Autodesk Fusion 360 part; units mm, degrees
sketch "Sketch1" plane through (0, 0, 0) normal (0, 0, 1) x (1, 0, 0)
  line L0 (10, -7.5) -> (-10, -7.5)
  line L1 (-10, -7.5) -> (-10, 7.5)
  line L2 (-10, 7.5) -> (10, 7.5)
  line L3 (10, 7.5) -> (10, -7.5)
  line L4 (10, -7.5) -> (-10, 7.5) construction
  line L5 (-10, -7.5) -> (10, 7.5) construction
  line L6 (0, 0) -> (0, 7) construction
  dimension "d1" = 20
  dimension "d2" = 15
extrude "Extrude1" add sketch "Sketch1" along normal blind 4
sketch "Sketch2" plane through (0, 0, 4) normal (0, 0, 1) x (-1, 0, 0)
  line L0 (-10, -7.5) -> (10, -7.5)
  line L1 (10, -7.5) -> (10, 7.5)
  line L2 (10, 7.5) -> (-10, 7.5)
  line L3 (-10, 7.5) -> (-10, -7.5)
  line L4 (10, 7.5) -> (-10, -7.5) construction
  line L5 (-10, 7.5) -> (10, -7.5) construction
  line L6 (0, 0) -> (-3, 0) construction
  circle A0 centre (-3, 0) radius 1
  line L7 (0, 0) -> (3, 0) construction
  circle A1 centre (3, 0) radius 1
  dimension "d5" = 3
  dimension "d6" = 2
  dimension "d7" = 3
  dimension "d8" = 2
extrude "Extrude2" cut sketch "Sketch2" against normal up to surface (4 mm away) contours A0 | A1
ref_plane "WorkPlane1" through (48, 0, 2) normal (1, 0, 0) x (0, 1, 0)
sketch "Sketch3" plane through (48, 0, 2) normal (1, 0, 0) x (0, 1, 0)
  line L0 (-7.5, 2) -> (-2.5, 2)
  line L1 (-2.5, 2) -> (-2.5, -2)
  line L2 (-2.5, -2) -> (-7.5, -2)
  line L3 (-7.5, -2) -> (-7.5, 2)
  line L4 (7.5, 2) -> (2.5, 2)
  line L5 (2.5, 2) -> (2.5, -2)
  line L6 (2.5, -2) -> (7.5, -2)
  line L7 (7.5, -2) -> (7.5, 2)
extrude "Extrude3" add sketch "Sketch3" against normal up to surface (38 mm away)
sketch "Sketch4" plane through (0, -2.5, 0) normal (0, 1, 0) x (-1, 0, 0)
  line L0 (-10, 0) -> (-10, 4)
  line L1 (-10, 4) -> (-48, 4)
  line L2 (-48, 4) -> (-48, 0)
  line L3 (-48, 0) -> (-10, 0)
  line L4 (-48, 4) -> (-44, 4)
  line L5 (-44, 4) -> (-44, 0)
  line L6 (-44, 0) -> (-48, 0)
  line L7 (-48, 0) -> (-48, 4)
extrude "Extrude4" add sketch "Sketch4" along normal up to surface (5 mm away) contours L1 L2 L3 L4 L5 L6 L7
sketch "Sketch5" plane through (0, 0, 4) normal (0, 0, 1) x (-1, 0, 0)
  line L0 (-44, 2.5) -> (-10, 2.5)
  line L1 (-10, 2.5) -> (-10, -2.5)
  line L2 (-10, -2.5) -> (-44, -2.5)
  line L3 (-44, -2.5) -> (-44, 2.5)
  circle A0 centre (3, 0) radius 1
  circle A1 centre (-3, 0) radius 1
  line L4 (-48, 7.5) -> (-48, -7.5)
  line L5 (-48, -7.5) -> (10, -7.5)
  line L6 (10, -7.5) -> (10, 7.5)
  line L7 (10, 7.5) -> (-48, 7.5)
  line L8 (-44, -2.5) -> (-44, -7.5)
  line L9 (-44, 2.5) -> (-44, 7.5)
extrude "Extrude5" add sketch "Sketch5" along normal blind 13 contours L3 L4 L5 L7 L8 L9
ref_plane "WorkPlane2" through (-48, 0, 2) normal (-1, 0, 0) x (0, -1, 0)
sketch "Sketch6" plane through (-48, 0, 2) normal (-1, 0, 0) x (0, 1, 0)
  line L0 (7.5, -2) -> (2.5, -2)
  line L1 (2.5, -2) -> (2.5, 2)
  line L2 (2.5, 2) -> (7.5, 2)
  line L3 (7.5, 2) -> (7.5, -2)
  line L4 (-7.5, -2) -> (-2.5, -2)
  line L5 (-2.5, -2) -> (-2.5, 2)
  line L6 (-2.5, 2) -> (-7.5, 2)
  line L7 (-7.5, 2) -> (-7.5, -2)
extrude "Extrude6" add sketch "Sketch6" against normal up to surface (38 mm away)
sketch "Sketch7" plane through (0, 2.5, 0) normal (0, -1, 0) x (1, 0, 0)
  line L0 (-10, 0) -> (-10, 4)
  line L1 (-10, 4) -> (-48, 4)
  line L2 (-48, 4) -> (-48, 0)
  line L3 (-48, 0) -> (-10, 0)
  line L4 (-48, 4) -> (-44, 4)
  line L5 (-44, 4) -> (-44, 0)
  line L6 (-44, 0) -> (-48, 0)
  line L7 (-48, 0) -> (-48, 4)
extrude "Extrude7" add sketch "Sketch7" along normal up to surface (5 mm away) contours L1 L2 L3 L4 L5 L6 L7
sketch "Sketch8" plane through (0, 0, 4) normal (0, 0, 1) x (-1, 0, 0)
  line L0 (44, -2.5) -> (10, -2.5)
  line L1 (10, -2.5) -> (10, 2.5)
  line L2 (10, 2.5) -> (44, 2.5)
  line L3 (44, 2.5) -> (44, -2.5)
  circle A0 centre (-3, 0) radius 1
  circle A1 centre (3, 0) radius 1
  line L4 (48, -7.5) -> (48, 7.5)
  line L5 (48, 7.5) -> (-44, 7.5)
  line L6 (-44, 7.5) -> (-44, 2.5)
  line L7 (-44, 2.5) -> (-10, 2.5)
  line L8 (-10, 2.5) -> (-10, -2.5)
  line L9 (-10, -2.5) -> (-44, -2.5)
  line L10 (-44, -2.5) -> (-44, -7.5)
  line L11 (-44, -7.5) -> (48, -7.5)
  line L12 (44, 2.5) -> (44, 7.5)
  line L13 (44, -2.5) -> (44, -7.5)
extrude "Extrude8" add sketch "Sketch8" along normal blind 13 contours L3 L4 L5 L11 L12 L13
For this review, take the finished solid that the model builds, in its own axes (mm). A direction names the side the tool comes from. Round coordinates to 2 decimals unless told otherwise and drop trailing zeros. Order: outer loops, then holes, each group sorted by start corner. A loop starts at its lowest first (then second) coordinate and runs counter-clockwise, first axis right, second up. Notation, with made-up numbers: (-9, 45) -> (35, 45) arc R11 cw to (35, 60) -> close; hole circle Ø3 at (20, 89). An arc over 180 degrees is marked (long way). Write item = value, one per line. Start each with the question number.
1) Take a section at A-A on x = -3. State the section outline as (y, z) points.
2) Tool access review of faces 5 (the face through (-46, 0, 17)), 6 (the face through (-27, -2.5, 2)): name each direction out of +Z, -Z, +X, -X, +Y, -Y from which nothing blocks a thin tool from reaching the whole face with its end or side.
3) Take a section at C-C on y = 0. State the section outline as (x, z) points.
4) Take a section at D-D on z = 8.25. State the section outline as (x, y) points, plus the area to 3 significant figures.
5) The part is to be moulded in two halves that separate along X. For faces 1 (the face through (48, 0, 8)), 2 (the face through (1, 0, 4)), 3 (the face through (10, 0, 2)), 4 (the face through (0, -7.5, 3)), say which applies: +X half, -X half, draft (parallel to the pull), parting line (faces both ways), or undercut.
6) Insertion check: pin 1 (8 mm diameter, centred on x = -26.5, z = 6, fed in from -Y); pin 2 (8 mm diameter, centred on x = -29.5, y = -1, fed in from +Z). Each pin has a flat end and moves straight along its axis. Give the tip position at first contact, or say it passes through.
7) Take a section at B-B on z = 1.75. State the section outline as (x, y) points.
8) To check wall thickness, follow line 1 (Y direction, x = -3, z = 1.2); line 2 (X direction, y = 1.5, z = 4.25); line 3 (Y direction, x = 23.5, z = 2.5). State the ranges of each line that lie inside material, in increasing order. Write a range as from..to.
Verdict:
q1.outline = (-7.5, 0) -> (-1, 0) -> (-1, 4) -> (-7.5, 4) -> close; (1, 0) -> (7.5, 0) -> (7.5, 4) -> (1, 4) -> close
q2.face_5 = +Z, +X, -X, +Y, -Y
q2.face_6 = +Z, -Z
q3.outline = (-48, 0) -> (-44, 0) -> (-44, 17) -> (-48, 17) -> close; (-10, 0) -> (-4, 0) -> (-4, 4) -> (-10, 4) -> close; (-2, 0) -> (2, 0) -> (2, 4) -> (-2, 4) -> close; (4, 0) -> (10, 0) -> (10, 4) -> (4, 4) -> close; (44, 0) -> (48, 0) -> (48, 17) -> (44, 17) -> close
q4.outline = (-48, -7.5) -> (-44, -7.5) -> (-44, 7.5) -> (-48, 7.5) -> close; (44, -7.5) -> (48, -7.5) -> (48, 7.5) -> (44, 7.5) -> close
q4.area = 120 mm2
q5.face_1 = +X half
q5.face_2 = undercut
q5.face_3 = undercut
q5.face_4 = draft
q6.pin_1 = -7.5
q6.pin_2 = 4
q7.outline = (-48, -7.5) -> (48, -7.5) -> (48, 7.5) -> (-48, 7.5) -> close; hole (-44, -2.5) -> (-10, -2.5) -> (-10, 2.5) -> (-44, 2.5) -> close; hole circle Ø2 at (-3, 0); hole circle Ø2 at (3, 0); hole (10, -2.5) -> (44, -2.5) -> (44, 2.5) -> (10, 2.5) -> close
q8.line_1 = -7.5..-1, 1..7.5
q8.line_2 = -48..-44, 44..48
q8.line_3 = -7.5..-2.5, 2.5..7.5
